Geometry: final body of the model. Coordinates: model frame, mm. Face numbers are marked on the shaded views. A direction names the side the tool comes from. Give positions to 0.01 mm unless a question says otherwise; leave off trailing zeros. Loops run counter-clockwise (first coordinate to the right, second up) from the corner with the lowest first, then second, coordinate; pieces in that order, holes last. Notation, with made-up numbers: (33.25, -17.75) -> (37.25, -17.75) arc R33 cw to (37.25, 20.25) -> close; hole circle Ø3 at (84, -24.5). An arc over 180 degrees is marked (long way). Answer in a Markdown table with one row per item. Add a question column.
1) First-contact query: P1, Ø6, axis at x = 15.5, y = -180, coming from the +Z side; P2, Ø6, axis at x = 64, z = 12, coming from the +Y side; P3, Ø10, axis at x = 235.5, z = 684.5, coming from the +Y side. Flat tips, straight axial feed; report the tip coordinate or a pass-through.
2) Line query: line 1 (Z direction, x = -127, y = 201.5); line 2 (Z direction, x = 201.5, y = 261); line 3 (Z direction, x = -123.5, y = -45.5). Output: solid intervals per line, ascending. Write a range as from..to.
3) Section query D-D (z = 803.5). Return the cut outline in (x, y), plus the area to 3 significant figures.
4) Access query for the marked faces 1 and 2. Directions: +Z, -Z, +X, -X, +Y, -Y. A direction counts if a zero-diameter tool reaches every point of the face in a straight line with its end or side. Return the directions, or none.
5) Section query A-A (y = 113). Return the cut outline in (x, z), plus the area to 3 significant figures.
6) Section query C-C (x = -200). Return the cut outline in (y, z), plus the area to 3 significant figures.
7) Draft query along Z for the marked faces 3, 4 and 5. Return one class per face: +Z half, -Z half, draft (parallel to the pull), parting line (faces both ways), or undercut.
8) Section query B-B (y = -12). Return the cut outline in (x, z), plus the area to 3 significant figures.
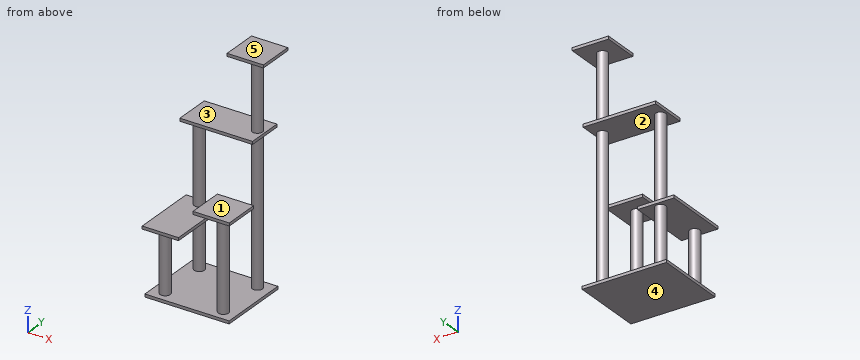
```python
from build123d import *

# Parameters (mm, degrees)
F0_W      = 580
F0_H      = 500
F1_DEPTH  = 20
F2_R      = 35
F3_DEPTH  = 400
F4_W      = 250
F4_H      = 450
F5_DEPTH  = 20
F6_DEPTH  = 1000
F7_R      = 35
F8_DEPTH  = 580
F9_DEPTH  = 650
F10_W     = 250
F10_H     = 250
F10_R     = 35
F11_DEPTH = 20
F12_W     = 500
F12_H     = 250
F13_DEPTH = 20
F14_R     = 35
F15_DEPTH = 500
F16_W     = 250
F16_H     = 250
F17_DEPTH = 20


with BuildPart() as f1:
    # F0 (on Top) → F1 (new body)
    with BuildSketch(Plane.XY):
        Rectangle(F0_W, F0_H)
    extrude(amount=F1_DEPTH)

    # F2 (on face) → F3 (join)
    with BuildSketch(Plane.XY.offset(20)):
        with Locations((-200, 175)):
            Circle(F2_R)
        with Locations((-200, -175)):
            Circle(F2_R)
    extrude(amount=F3_DEPTH)

    # F4 (on face) → F5 (join)
    with BuildSketch(Plane.XY.offset(420)):
        with Locations((-200, 0)):
            Rectangle(F4_W, F4_H)
    extrude(amount=F5_DEPTH)

    # F2 (on face) → F6 (join)
    with BuildSketch(Plane.XY.offset(20)):
        with Locations((200, 175)):
            Circle(F2_R)
    extrude(amount=F6_DEPTH)

    # F7 (on face) → F8 (join, through all)
    with BuildSketch(Plane.XY.offset(440)):
        with Locations((-200, 175)):
            Circle(F7_R)
    extrude(amount=F8_DEPTH)

    # F2 (on face) → F9 (join)
    with BuildSketch(Plane.XY.offset(20)):
        with Locations((200, -175)):
            Circle(F2_R)
    extrude(amount=F9_DEPTH)

    # F10 (on face) → F11 (join)
    with BuildSketch(Plane.XY.offset(670)):
        with Locations((200, -175)):
            Rectangle(F10_W, F10_H)
        with Locations((200, -175)):
            Circle(F10_R, mode=Mode.SUBTRACT)
        with Locations((200, -175)):
            Circle(F10_R)
    extrude(amount=F11_DEPTH)

    # F12 (on face) → F13 (join)
    with BuildSketch(Plane.XY.offset(1020)):
        with Locations((0, 175)):
            Rectangle(F12_W, F12_H)
    extrude(amount=F13_DEPTH)

    # F14 (on face) → F15 (join)
    with BuildSketch(Plane.XY.offset(1040)):
        with Locations((200, 175)):
            Circle(F14_R)
    extrude(amount=F15_DEPTH)

    # F16 (on face) → F17 (join)
    with BuildSketch(Plane.XY.offset(1540)):
        with Locations((200, 175)):
            Rectangle(F16_W, F16_H)
    extrude(amount=F17_DEPTH)


solid = f1.part
```
Evaluation:
| question | item | result |
|---|---|---|
| 1 | P1 | z = 20 |
| 1 | P2 | y = 250 |
| 1 | P3 | y = 192.17 |
| 2 | line 1 | 0..20, 420..440, 1020..1040 |
| 2 | line 2 | 1020..1040, 1540..1560 |
| 2 | line 3 | 0..20, 420..440 |
| 3 | outline | circle Ø70 at (-200, 175); circle Ø70 at (200, 175) |
| 3 | area | 7,700 mm² |
| 4 | face 1 | +Z, +X, -X, -Y |
| 4 | face 2 | none |
| 5 | outline | (-325, 420) -> (-75, 420) -> (-75, 440) -> (-325, 440) -> close; (-290, 0) -> (290, 0) -> (290, 20) -> (-290, 20) -> close; (-250, 1020) -> (250, 1020) -> (250, 1040) -> (-250, 1040) -> close; (75, 1540) -> (325, 1540) -> (325, 1560) -> (75, 1560) -> close |
| 5 | area | 31,600 mm² |
| 6 | outline | (-250, 0) -> (250, 0) -> (250, 20) -> (210, 20) -> (210, 420) -> (225, 420) -> (225, 440) -> (210, 440) -> (210, 1020) -> (300, 1020) -> (300, 1040) -> (50, 1040) -> (50, 1020) -> (140, 1020) -> (140, 440) -> (-225, 440) -> (-225, 420) -> (-210, 420) -> (-210, 20) -> (-250, 20) -> close; hole (-140, 20) -> (140, 20) -> (140, 420) -> (-140, 420) -> close |
| 6 | area | 121,000 mm² |
| 7 | face 3 | undercut |
| 7 | face 4 | -Z half |
| 7 | face 5 | +Z half |
| 8 | outline | (-325, 420) -> (-75, 420) -> (-75, 440) -> (-325, 440) -> close; (-290, 0) -> (290, 0) -> (290, 20) -> (-290, 20) -> close |
| 8 | area | 16,600 mm² |
